```python
from build123d import *

# Parameters (mm, degrees)
SKETCH1_W           = 500
SKETCH1_H           = 800
BOSS_EXTRUDE1_DEPTH = 10
CUT_EXTRUDE1_DEPTH  = 10


with BuildPart() as part:
    # Sketch1 → Boss-Extrude1 (new body)
    with BuildSketch(Plane(origin=(0, 0, 0), x_dir=(1, 0, 0), z_dir=(0, 1, 0))):
        Rectangle(SKETCH1_W, SKETCH1_H)
    extrude(amount=BOSS_EXTRUDE1_DEPTH)

    # Sketch2 → Cut-Extrude1 (cut)
    with BuildSketch(Plane(origin=(0, 10, 0), x_dir=(1, 0, 0), z_dir=(0, 1, 0))):
        Polygon((-160, -70), (-210, -70), (-210, 70), (-160, 70), (-160, 20), (-110, 20), (-110, -20), (-160, -20), align=None)
    cut_extrude1 = extrude(amount=-CUT_EXTRUDE1_DEPTH, mode=Mode.SUBTRACT)

    # Mirror1: Cut-Extrude1 across plane
    add(cut_extrude1.mirror(Plane(origin=(0, 0, 0), x_dir=(0, 0, 1), z_dir=(1, 0, 0))), mode=Mode.SUBTRACT)


solid = part.part
```
The listing builds one solid part. Answer for the finished solid, in the listing's coordinates (mm). Give positions to 0.01 mm unless a question says otherwise; leave off trailing zeros. Order: outer loops, then holes, each group sorted by start corner. A loop starts at its lowest first (then second) coordinate and runs counter-clockwise, first axis right, second up. Notation, with made-up numbers: (-4, 30.25) -> (24, 30.25) arc R14 ccw to (24, 57.25) -> close; hole circle Ø10 at (-20.5, 14.25). An arc over 180 degrees is marked (long way). Answer as CSV lines item,"result". Start each with the question number.
Q1. Find the intervals of material crossed by L1, parallel to X at y = 5, z = -2.5; L2, parallel to X at y = 8.25, z = 53; L3, parallel to Z at x = 208.5, y = 6.75, in increasing order.
Q2. A cutting plane is placed at B-B (z = 51). Determine the outline of the cut face in (x, y), then the cut area to 3 significant figures.
Q3. A cutting plane is placed at C-C (y = 7.75). Determine the outline of the cut face in (x, z), then the cut area to 3 significant figures.
Q4. Given pin 1 (10 mm diameter, centred on x = 171, z = 153, fed in from -Y), flat-ended and moving along its own axis, determine where the tip first touches the part or whether it passes through.
Q5. A cutting plane is placed at A-A (x = -152). Determine the outline of the cut face in (y, z), then the cut area to 3 significant figures.
Results found:
1,L1,"-250 to -210, -110 to 110, 210 to 250"
1,L2,"-250 to -210, -160 to 160, 210 to 250"
1,L3,"-400 to -70, 70 to 400"
2,outline,"(-250, 0) -> (-210, 0) -> (-210, 10) -> (-250, 10) -> close; (-160, 0) -> (160, 0) -> (160, 10) -> (-160, 10) -> close; (210, 0) -> (250, 0) -> (250, 10) -> (210, 10) -> close"
2,area,"4,000 mm2"
3,outline,"(-250, -400) -> (250, -400) -> (250, 400) -> (-250, 400) -> close; hole (-210, -70) -> (-160, -70) -> (-160, -20) -> (-110, -20) -> (-110, 20) -> (-160, 20) -> (-160, 70) -> (-210, 70) -> close; hole (110, -20) -> (160, -20) -> (160, -70) -> (210, -70) -> (210, 70) -> (160, 70) -> (160, 20) -> (110, 20) -> close"
3,area,"382,000 mm2"
4,pin 1,"y = 0"
5,outline,"(0, -400) -> (10, -400) -> (10, -20) -> (0, -20) -> close; (0, 20) -> (10, 20) -> (10, 400) -> (0, 400) -> close"
5,area,"7,600 mm2"
